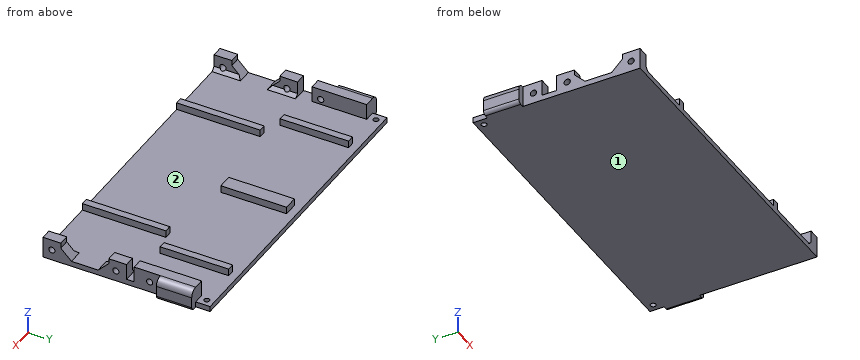
from build123d import *

# Parameters (mm, degrees)
SKETCH_1_W          = 180
SKETCH_1_H          = 94
EXTRUDE_1_DEPTH     = 3
SKETCH_2_W          = 6
SKETCH_2_H          = 10
SKETCH_2_H_2        = 34.6
SKETCH_2_H_3        = 30.754035876
EXTRUDE_2_DEPTH     = 9
CHAMFER_2_SIZE      = 6
CHAMFER_1_SIZE      = 6
SKETCH_3_R          = 1.75
CUT_EXTRUDE_1_DEPTH = 204.420746238
SKETCH_4_R          = 1.5
CUT_EXTRUDE_2_DEPTH = 204.265835791
SKETCH_5_W          = 4
SKETCH_5_H          = 47
SKETCH_5_H_2        = 38.5
SKETCH_5_W_2        = 8
SKETCH_5_H_3        = 37
EXTRUDE_3_DEPTH     = 4
CHAMFER_3_SIZE      = 2
SKETCH_6_W          = 12
SKETCH_6_H          = 19.9
EXTRUDE_4_DEPTH     = 4
FILLET_1_R          = 4
SKETCH_7_W          = 12
SKETCH_7_H          = 19.9
EXTRUDE_5_DEPTH     = 4
FILLET_2_R          = 4
FILLET_3_R          = 2


with BuildPart() as part:
    # Эскиз1 → Бобышка-Вытянуть1 (new body)
    with BuildSketch(Plane.XY):
        with Locations((90, -47)):
            Rectangle(SKETCH_1_W, SKETCH_1_H)
    extrude(amount=EXTRUDE_1_DEPTH)

    # Эскиз2 → Бобышка-Вытянуть2 (add)
    with BuildSketch(Plane.XY.offset(3)):
        with Locations((3, -89)):
            Rectangle(SKETCH_2_W, SKETCH_2_H)
        with Locations((177, -89)):
            Rectangle(SKETCH_2_W, SKETCH_2_H)
        with Locations((3, -52)):
            Rectangle(SKETCH_2_W, SKETCH_2_H)
        with Locations((177, -52)):
            Rectangle(SKETCH_2_W, SKETCH_2_H)
        with Locations((177, -25.4)):
            Rectangle(SKETCH_2_W, SKETCH_2_H_2)
        with Locations((3, -23.477017938)):
            Rectangle(SKETCH_2_W, SKETCH_2_H_3)
    extrude(amount=EXTRUDE_2_DEPTH)

    # Фаска2
    chamfer_2_edges = [part.edges().sort_by_distance(p)[0] for p in [
        (3, -57, 3),
        (177, -57, 3),
    ]]
    chamfer(chamfer_2_edges, length=CHAMFER_2_SIZE)

    # Фаска1
    chamfer_1_edges = [part.edges().sort_by_distance(p)[0] for p in [
        (3, -84, 3),
        (177, -84, 3),
    ]]
    chamfer(chamfer_1_edges, length=CHAMFER_1_SIZE)

    # Эскиз3 → Вырез-Вытянуть1 (cut, through all)
    with BuildSketch(Plane(origin=(180, 0, 0), x_dir=(0, 0, -1), z_dir=(1, 0, 0))):
        with Locations((-6, -89)):
            Circle(SKETCH_3_R)
        with Locations((-6, -53)):
            Circle(SKETCH_3_R)
        with Locations((-6, -34)):
            Circle(SKETCH_3_R)
    extrude(amount=-CUT_EXTRUDE_1_DEPTH, mode=Mode.SUBTRACT)

    # Эскиз4 → Вырез-Вытянуть2 (cut, through all)
    with BuildSketch(Plane.XY.offset(3)):
        with Locations((4, -4)):
            Circle(SKETCH_4_R)
        with Locations((176, -4)):
            Circle(SKETCH_4_R)
    extrude(amount=-CUT_EXTRUDE_2_DEPTH, mode=Mode.SUBTRACT)

    # Эскиз5 → Бобышка-Вытянуть3 (add)
    with BuildSketch(Plane.XY.offset(3)):
        with Locations((42, -70.5)):
            Rectangle(SKETCH_5_W, SKETCH_5_H)
        with Locations((138, -70.5)):
            Rectangle(SKETCH_5_W, SKETCH_5_H)
        with Locations((29, -23.75)):
            Rectangle(SKETCH_5_W, SKETCH_5_H_2)
        with Locations((151, -23.75)):
            Rectangle(SKETCH_5_W, SKETCH_5_H_2)
        with Locations((90, -23)):
            Rectangle(SKETCH_5_W_2, SKETCH_5_H_3)
    extrude(amount=EXTRUDE_3_DEPTH)

    # Фаска3
    # the kernel refuses this chamfer: 2 mm, written as the material it adds along each edge
    with BuildSketch(Plane(origin=(6, -72.856634024, 3), x_dir=(0.9996219169112968, 0, -0.02749587661058627), z_dir=(0, -1, 0))) as chamfer_3_piece_1_section:
        Polygon((CHAMFER_3_SIZE * 0.999621916911, CHAMFER_3_SIZE * 0.0274958766106), (-CHAMFER_3_SIZE * 0.0274958766106, CHAMFER_3_SIZE * 0.999621916911), (0, 0), align=None)
    chamfer_3_piece_1 = extrude(amount=21.143365976, mode=Mode.PRIVATE)
    chamfer_3_piece_1 = split(chamfer_3_piece_1, bisect_by=Plane(origin=(6.680922071, -82.46162584, 7.46162584), z_dir=(0, -0.7071067811865476, -0.7071067811865476)), keep=Keep.TOP, mode=Mode.PRIVATE)
    chamfer_3_piece_1 = chamfer_3_piece_1 - Plane(origin=(6.680922071, -89, 6), x_dir=(0, 0, -1), z_dir=(1, 0, 0)) * Cylinder(1.75, 51, mode=Mode.PRIVATE)
    add(chamfer_3_piece_1)
    with BuildSketch(Plane(origin=(174, -94, 3), x_dir=(-0.9996219169112968, 0, -0.02749587661058639), z_dir=(0, 1, 0))) as chamfer_3_piece_2_section:
        Polygon((CHAMFER_3_SIZE * 0.999621916911, CHAMFER_3_SIZE * 0.0274958766106), (-CHAMFER_3_SIZE * 0.0274958766106, CHAMFER_3_SIZE * 0.999621916911), (0, 0), align=None)
    chamfer_3_piece_2 = extrude(amount=21.143365976, mode=Mode.PRIVATE)
    chamfer_3_piece_2 = split(chamfer_3_piece_2, bisect_by=Plane(origin=(173.319077929, -82.46162584, 7.46162584), z_dir=(0, -0.7071067811865476, -0.7071067811865476)), keep=Keep.TOP, mode=Mode.PRIVATE)
    chamfer_3_piece_2 = chamfer_3_piece_2 - Plane(origin=(173.319077929, -89, 6), x_dir=(0, 0, -1), z_dir=(1, 0, 0)) * Cylinder(1.75, 51, mode=Mode.PRIVATE)
    add(chamfer_3_piece_2)
    with BuildSketch(Plane(origin=(6, -47, 3), x_dir=(0.9996219169112968, 0, -0.02749587661058627), z_dir=(0, -1, 0))) as chamfer_3_piece_3_section:
        Polygon((CHAMFER_3_SIZE * 0.999621916911, CHAMFER_3_SIZE * 0.0274958766106), (-CHAMFER_3_SIZE * 0.0274958766106, CHAMFER_3_SIZE * 0.999621916911), (0, 0), align=None)
    chamfer_3_piece_3 = extrude(amount=21.143365976, mode=Mode.PRIVATE)
    chamfer_3_piece_3 = split(chamfer_3_piece_3, bisect_by=Plane(origin=(6.680922071, -58.530709151, 7.469290849), z_dir=(0, 0.7071067811865476, -0.7071067811865476)), keep=Keep.TOP, mode=Mode.PRIVATE)
    chamfer_3_piece_3 = chamfer_3_piece_3 - Plane(origin=(6.680922071, -53, 6), x_dir=(0, 0, -1), z_dir=(1, 0, 0)) * Cylinder(1.75, 51, mode=Mode.PRIVATE)
    add(chamfer_3_piece_3)
    with BuildSketch(Plane(origin=(174, -68.143365976, 3), x_dir=(-0.9996219169112968, 0, -0.02749587661058639), z_dir=(0, 1, 0))) as chamfer_3_piece_4_section:
        Polygon((CHAMFER_3_SIZE * 0.999621916911, CHAMFER_3_SIZE * 0.0274958766106), (-CHAMFER_3_SIZE * 0.0274958766106, CHAMFER_3_SIZE * 0.999621916911), (0, 0), align=None)
    chamfer_3_piece_4 = extrude(amount=21.143365976, mode=Mode.PRIVATE)
    chamfer_3_piece_4 = split(chamfer_3_piece_4, bisect_by=Plane(origin=(173.319077929, -58.530709151, 7.469290849), z_dir=(0, 0.7071067811865476, -0.7071067811865476)), keep=Keep.TOP, mode=Mode.PRIVATE)
    chamfer_3_piece_4 = chamfer_3_piece_4 - Plane(origin=(173.319077929, -53, 6), x_dir=(0, 0, -1), z_dir=(1, 0, 0)) * Cylinder(1.75, 51, mode=Mode.PRIVATE)
    add(chamfer_3_piece_4)

    # Эскиз6 → Бобышка-Вытянуть4 (add)
    with BuildSketch(Plane(origin=(180, 0, 0), x_dir=(0, 0, -1), z_dir=(1, 0, 0))):
        with Locations((-6, -18.05)):
            Rectangle(SKETCH_6_W, SKETCH_6_H)
    extrude(amount=EXTRUDE_4_DEPTH)

    # Скругление1
    fillet_1_edges = [part.edges().sort_by_distance(p)[0] for p in [
        (184, -18.05, 12),
    ]]
    fillet(fillet_1_edges, radius=FILLET_1_R)

    # Эскиз7 → Бобышка-Вытянуть5 (add)
    with BuildSketch(Plane.ZY):
        with Locations((6, -18.05)):
            Rectangle(SKETCH_7_W, SKETCH_7_H)
    extrude(amount=EXTRUDE_5_DEPTH)

    # Скругление2
    fillet_2_edges = [part.edges().sort_by_distance(p)[0] for p in [
        (-4, -18.05, 12),
    ]]
    fillet(fillet_2_edges, radius=FILLET_2_R)

    # Скругление3
    fillet_3_edges = [part.edges().sort_by_distance(p)[0] for p in [
        (184, -18.05, 0),
        (-4, -18.05, 0),
    ]]
    fillet(fillet_3_edges, radius=FILLET_3_R)


solid = part.part
Check sheet for the modelled part. Datum: model origin and axes. Units: mm. Face numbers are marked on the shaded views. Round coordinates to 2 decimals unless told otherwise and drop trailing zeros. Order: outer loops, then holes, each group sorted by start corner. A loop starts at its lowest first (then second) coordinate and runs counter-clockwise, first axis right, second up. Notation, with made-up numbers: M 45.5,43 L 87.5,43 A16 cw 87.5,53 Z; hole C 42.5,-30 d9. An arc over 180 degrees is marked long. One line per item, written item: value. Start each with the question number.
1. Scan lines: line 1 along X through (y, z) = (-23.5, 5.25); line 2 along X through (y, z) = (-29.5, 4.5); line 3 along X through (y, z) = (-24, 7.75). Record each from-to range of solid material in increasing order.
2. Section check D-D on x = 60.5. Enter the section's corners in (y, z), and give its area (3 significant figures).
3. Gauge pin test, flat ends, axial feed: P1, Ø2, axis at x = 162.5, y = -55.5, coming from the +Z side; P2, Ø4.5, axis at x = 28.5, y = -29, coming from the +Z side; P3, Ø3, axis at y = -73, z = 4, coming from the -X side. Record the tip position at first contact, or that the pin passes through.
4. Release check for a two-part mould opening along X. For the marked faces 1 and 2 record: released by +X, released by -X, zero draft, split by the parting line, or undercut.
5. Section check A-A on y = -34. Enter the section's corners in (x, z).
6. Section check C-C on y = -10. Enter the section's corners in (x, z).
7. Section check B-B on y = -66. Enter the section's corners in (x, z).
Results found:
1. line 1: -4 to 6, 27 to 31, 86 to 94, 149 to 153, 174 to 184
1. line 2: 0 to 6, 27 to 31, 86 to 94, 149 to 153, 174 to 180
1. line 3: -4 to 6, 174 to 184
2. outline: M -94,0 L 0,0 L 0,3 L -94,3 Z
2. area: 282 mm^2
3. P1: z = 3
3. P2: z = 7
3. P3: x = 0
4. face 1: zero draft
4. face 2: undercut
5. outline: M 0,0 L 180,0 L 180,4.25 L 174,4.25 L 174,3 L 153,3 L 153,7 L 149,7 L 149,3 L 94,3 L 94,7 L 86,7 L 86,3 L 31,3 L 31,7 L 27,7 L 27,3 L 6,3 L 6,4.25 L 0,4.25 Z; M 0,7.75 L 6,7.75 L 6,12 L 0,12 Z; M 174,7.75 L 180,7.75 L 180,12 L 174,12 Z
6. outline: M -4,2 A2 ccw -2,0 L 182,0 A2 ccw 184,2 L 184,8 A4 ccw 180,12 L 174,12 L 174,3 L 153,3 L 153,7 L 149,7 L 149,3 L 94,3 L 94,7 L 86,7 L 86,3 L 31,3 L 31,7 L 27,7 L 27,3 L 6,3 L 6,12 L 0,12 A4 ccw -4,8 Z
7. outline: M 0,0 L 180,0 L 180,3 L 140,3 L 140,7 L 136,7 L 136,3 L 44,3 L 44,7 L 40,7 L 40,3 L 0,3 Z
